```python
from build123d import *

# Parameters (mm, degrees)
F0_W      = 96
F0_H      = 86
F1_DEPTH  = 66
F3_D      = 28
F5_D      = 28
F7_D      = 8.8
F7_DEPTH  = 20
F7_TIP    = 2.6437867237
F9_D      = 6.6
F9_DEPTH  = 20
F9_TIP    = 1.9828400428
F11_D     = 6.6
F11_DEPTH = 20
F11_TIP   = 1.9828400428
F13_D     = 6.6
F13_DEPTH = 20
F13_TIP   = 1.9828400428
F15_D     = 6.6
F15_DEPTH = 20
F15_TIP   = 1.9828400428


with BuildPart() as f1:
    # F0 (on Front) → F1 (new body)
    with BuildSketch(Plane.XZ):
        with Locations((48, -43)):
            Rectangle(F0_W, F0_H)
    extrude(amount=-F1_DEPTH)

    # F3 (through all)
    with Locations(Plane.XY):
        with Locations((18, 18), (78, 18)):
            Hole(F3_D / 2)

    # F5 (through all)
    with Locations(Plane.YZ.offset(96)):
        with Locations((48, -23), (48, -63)):
            Hole(F5_D / 2)

    # F7
    with Locations(Plane.XY):
        with Locations((48, 18)):
            Hole(F7_D / 2, depth=F7_DEPTH)
            with Locations((0, 0, -(F7_DEPTH + F7_TIP / 2))):  # 118° drill point
                Cone(0, F7_D / 2, F7_TIP, mode=Mode.SUBTRACT)

    # F9
    with Locations(Plane.XY):
        with Locations((32, 31)):
            Hole(F9_D / 2, depth=F9_DEPTH)
            with Locations((0, 0, -(F9_DEPTH + F9_TIP / 2))):  # 118° drill point
                Cone(0, F9_D / 2, F9_TIP, mode=Mode.SUBTRACT)

    # F11
    with Locations(Plane.YZ.offset(96)):
        with Locations((48, -81), (48, -5)):
            Hole(F11_D / 2, depth=F11_DEPTH)
            with Locations((0, 0, -(F11_DEPTH + F11_TIP / 2))):  # 118° drill point
                Cone(0, F11_D / 2, F11_TIP, mode=Mode.SUBTRACT)

    # F13
    with Locations(Plane(origin=(0, 0, -86), x_dir=(1, 0, 0), z_dir=(0, 0, -1))):
        with Locations((32, -31)):
            Hole(F13_D / 2, depth=F13_DEPTH)
            with Locations((0, 0, -(F13_DEPTH + F13_TIP / 2))):  # 118° drill point
                Cone(0, F13_D / 2, F13_TIP, mode=Mode.SUBTRACT)

    # F15
    with Locations(Plane(origin=(0, 0, 0), x_dir=(0, -1, 0), z_dir=(-1, 0, 0))):
        with Locations((-56, -46), (-40, -40)):
            Hole(F15_D / 2, depth=F15_DEPTH)
            with Locations((0, 0, -(F15_DEPTH + F15_TIP / 2))):  # 118° drill point
                Cone(0, F15_D / 2, F15_TIP, mode=Mode.SUBTRACT)


solid = f1.part
```
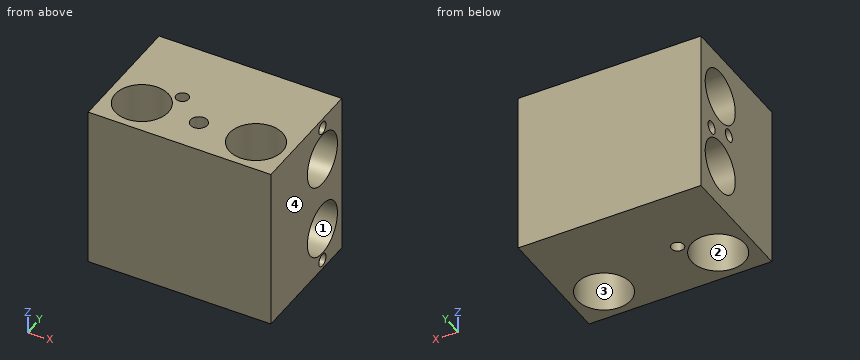
Work out the finished part from the listing and answer in its coordinate system (mm). Face numbers are marked on the shaded views. Coordinates: 2 decimals unless noted, no trailing zeros. Loops run counter-clockwise (first coordinate to the right, second up) from the corner with the lowest first, then second, coordinate; pieces in that order, holes last. Notation, with made-up numbers: (-35, 16.5) -> (-16, 16.5) arc R26 cw to (-16, 39.5) -> close; hole circle Ø10 at (73, 77). An arc over 180 degrees is marked (long way). Answer as CSV lines item,"result".
Q1. The part is cut by section D-D on y = 7. Write down the section's boundary in (x, z).
Findings:
outline,"(0, -86) -> (9.34, -86) -> (9.34, 0) -> (0, 0) -> close; (26.66, -86) -> (69.34, -86) -> (69.34, 0) -> (26.66, 0) -> close; (86.66, -86) -> (96, -86) -> (96, 0) -> (86.66, 0) -> close"
Q2. The part is cut by section C-C on z = -72.5. Write down the section's boundary in (x, y).
Findings:
outline,"(0, 0) -> (96, 0) -> (96, 37.72) -> (0, 37.72) -> close; (0, 58.28) -> (96, 58.28) -> (96, 66) -> (0, 66) -> close; hole circle Ø28 at (18, 18); hole circle Ø6.6 at (32, 31); hole circle Ø28 at (78, 18)"
Q3. The part is cut by section A-A on z = -15.5. Write down the section's boundary in (x, y).
Findings:
outline,"(0, 0) -> (96, 0) -> (96, 36.18) -> (0, 36.18) -> close; (0, 59.82) -> (96, 59.82) -> (96, 66) -> (0, 66) -> close; hole circle Ø28 at (18, 18); hole circle Ø6.6 at (32, 31); hole circle Ø8.8 at (48, 18); hole circle Ø28 at (78, 18)"
Q4. Find the intervals of material crossed by probe 1 along Z at (x, y) = (27, 48); probe 2 along Y at (x, z) = (92.25, -5); probe 3 along Y at (x, z) = (10.5, -35.5), in increasing order.
Findings:
probe 1,"z = -86 to -77, -49 to -37, -9 to 0"
probe 2,"y = 0 to 44.7, 51.3 to 66"
probe 3,"y = 0 to 6.18, 29.82 to 41.7, 54.3 to 66"
Q5. The part is cut by section B-B on x = 40. Write down the section's boundary in (y, z), and give its area (3 significant figures).
Findings:
outline,"(0, -86) -> (66, -86) -> (66, 0) -> (0, 0) -> close; hole circle Ø28 at (48, -63); hole circle Ø28 at (48, -23)"
area,"4,440 mm²"
Q6. For a pull along X with two mould halves and no side action, classify the marked faces 1, 2, 3 and 4 as +X half, -X half, draft (parallel to the pull), parting line (faces both ways), or undercut.
Findings:
face 1,"draft"
face 2,"undercut"
face 3,"undercut"
face 4,"+X half"
Q7. Each of these flat-tipped pins is pushed along its axis until it touches: pin 1 (5.5 mm diameter, centred on x = 32, y = 31, fed in from -Z); pin 2 (4 mm diameter, centred on y = 56, z = -46, fed in from -X); pin 3 (4 mm diameter, centred on y = 48, z = -5, fed in from +X). Where does it stop, or does it pass through?
Findings:
pin 1,"stops at z = -65.67"
pin 2,"stops at x = 20.78"
pin 3,"stops at x = 75.22"
